```python
from build123d import *

# Parameters (mm, degrees)
F0_W     = 457.2
F0_H     = 914.4
F0_W_2   = 101.6
F0_H_2   = 171.45
F1_DEPTH = 6.35
F2_W     = 381
F2_H     = 38.1
F2_W_2   = 266.7
F2_W_3   = 38.1
F2_H_2   = 187.325
F3_DEPTH = 139.7
F4_W     = 193.675
F4_H     = 6.35
F5_DEPTH = 165.1
F6_W     = 304.8
F6_H     = 254
F7_DEPTH = 12.7
F9_DEPTH = 254
F11_D    = 3.175


with BuildPart() as f1:
    # F0 (on Top) → F1 (new body)
    with BuildSketch(Plane.XY):
        Rectangle(F0_W, F0_H)
        with Locations((133.35, 271.4625)):
            Rectangle(F0_W_2, F0_H_2, mode=Mode.SUBTRACT)
    extrude(amount=F1_DEPTH)

    # F2 (on face) → F3 (join)
    with BuildSketch(Plane(origin=(0, 0, 0), x_dir=(1, 0, 0), z_dir=(0, 0, -1))):
        Polygon((-190.5, 457.2), (-228.6, 457.2), (-228.6, -457.2), (-190.5, -457.2), (-190.5, -419.1), align=None)
        with Locations((0, -438.15)):
            Rectangle(F2_W, F2_H)
        Polygon((190.5, -403.225), (190.5, -419.1), (190.5, -457.2), (228.6, -457.2), (228.6, -368.3), (190.5, -368.3), align=None)
        Polygon((228.6, -174.625), (228.6, 203.2), (190.5, 203.2), (190.5, 165.1), (190.5, -139.7), (190.5, -174.625), align=None)
        with Locations((57.15, 184.15)):
            Rectangle(F2_W_2, F2_H)
        Polygon((28.575, -403.225), (190.5, -403.225), (190.5, -368.3), (190.5, -365.125), (66.675, -365.125), (28.575, -365.125), align=None)
        with Locations((47.625, -271.4625)):
            Rectangle(F2_W_3, F2_H_2)
        Polygon((190.5, -177.8), (190.5, -174.625), (190.5, -139.7), (28.575, -139.7), (28.575, -177.8), (66.675, -177.8), align=None)
    extrude(amount=F3_DEPTH)

    # F4 (on face) → F5 (cut)
    with BuildSketch(Plane.YZ.offset(228.6)):
        with Locations((271.4625, -76.2)):
            Rectangle(F4_W, F4_H)
    extrude(amount=-F5_DEPTH, mode=Mode.SUBTRACT)

    # F6 (on face) → F7 (cut)
    with BuildSketch(Plane.XY.offset(6.35)):
        with Locations((76.2, -330.2)):
            Rectangle(F6_W, F6_H)
    extrude(amount=-F7_DEPTH, mode=Mode.SUBTRACT)

    # F8 (on face) → F9 (join)
    with BuildSketch(Plane.XZ.offset(203.2)):
        Polygon((228.6, -132.720256), (-76.2, 6.35), (-76.2, 0), (-76.2, -0.629744), (228.6, -139.7), align=None)
    extrude(amount=F9_DEPTH)

    # F11 (through all)
    with Locations(Plane.XY.offset(6.35)):
        with Locations((222.25, 336.55), (222.25, 323.85), (222.25, 219.075), (222.25, 206.375)):
            Hole(F11_D / 2)


solid = f1.part
```
Build history of the part. All positions in model axes, mm. A direction names the side the tool comes from. Give positions to 0.01 mm unless a question says otherwise; leave off trailing zeros. Loops run counter-clockwise (first coordinate to the right, second up) from the corner with the lowest first, then second, coordinate; pieces in that order, holes last. Notation, with made-up numbers: (49, -39.75) - (83, -39.75) arc R20 ccw to (83, -31.75) - close; hole circle Ø3 at (52, -29.75). An arc over 180 degrees is marked (long way). Use a Markdown table: item, result.
(1) Wall check: line 1 along Y through (x, z) = (222.25, 3.5); line 2 along X through (y, z) = (336.55, 5); line 3 along Y through (x, z) = (222, 2). Give the ranges that are in metal, low to high.
Taken from the geometry:
| item | result |
|---|---|
| line 1 | -203.2 to 204.79, 207.96 to 217.49, 220.66 to 322.26, 325.44 to 334.96, 338.14 to 457.2 |
| line 2 | -228.6 to 82.55, 184.15 to 220.66, 223.84 to 228.6 |
| line 3 | -203.2 to 204.81, 207.94 to 217.51, 220.64 to 322.28, 325.42 to 334.98, 338.12 to 457.2 |
(2) Band-saw the part on D-D (z = -16.5). Give the cut face in (x, y) (3 decimals), and give its area (3 significant figures).
Taken from the geometry:
| item | result |
|---|---|
| outline | (-228.6, -457.2) - (-190.5, -457.2) - (-190.5, 419.1) - (190.5, 419.1) - (190.5, 403.225) - (28.575, 403.225) - (28.575, 139.7) - (190.5, 139.7) - (190.5, -165.1) - (-76.2, -165.1) - (-76.2, -203.2) - (-41.417, -203.2) - (-41.417, -457.2) - (-26.12, -457.2) - (-26.12, -203.2) - (228.6, -203.2) - (228.6, 174.625) - (190.5, 174.625) - (190.5, 177.8) - (66.675, 177.8) - (66.675, 365.125) - (190.5, 365.125) - (190.5, 368.3) - (228.6, 368.3) - (228.6, 457.2) - (-228.6, 457.2) - close |
| area | 101,000 mm2 |
(3) Pull direction X, two halves, no side cores. Call faces 1 (the face through (66.675, 273, -109)), 2 (the face through (-3, 419.1, -69)), 3 (the face through (-137, -457.2, 4)): +X half, -X half, draft (parallel to the pull), parting line (faces both ways), or undercut.
Taken from the geometry:
| item | result |
|---|---|
| face 1 | +X half |
| face 2 | undercut |
| face 3 | draft |
(4) Drop flat-ended pins along their axis: pin 1 Ø12 at (x, z) = (-150, -73.5) entering from -Y; pin 2 Ø1 at (y, z) = (366, -116.5) entering from +X; pin 3 Ø10 at (x, y) = (95, 101) entering from -Z. Give the stop position or say it passes through.
Taken from the geometry:
| item | result |
|---|---|
| pin 1 | y = 419.1 |
| pin 2 | x = 190.5 |
| pin 3 | z = 0 |
(5) Band-saw the part on B-B (y = 35). Give the cut face in (x, z), and give its area (3 significant figures).
Taken from the geometry:
| item | result |
|---|---|
| outline | (-228.6, -139.7) - (-190.5, -139.7) - (-190.5, 0) - (190.5, 0) - (190.5, -139.7) - (228.6, -139.7) - (228.6, 6.35) - (-228.6, 6.35) - close |
| area | 13,500 mm2 |
(6) Which spindle directions (+Z, -Z, +X, -X, +Y, -Y) get a long thin tool onto all of the face, cutting with end or side? Do faces 4 (the face through (28.575, 270, -69)), 5 (the face through (66, 228, -79.375)), 6 (the face through (78.334, -328.422, -64.159)), 7 (the face through (129, 365.125, -109)), 8 (the face through (6, -203.2, -100)). Say none if no direction does.
Taken from the geometry:
| item | result |
|---|---|
| face 4 | -Z |
| face 5 | +X |
| face 6 | +Z, +X, -Y |
| face 7 | -Z, +X |
| face 8 | -Z, -Y |
(7) Band-saw the part on A-A (y = 271.5). Give the cut face in (x, z) (3 decimals).
Taken from the geometry:
| item | result |
|---|---|
| outline | (-228.6, -139.7) - (-190.5, -139.7) - (-190.5, 0) - (28.575, 0) - (28.575, -139.7) - (66.675, -139.7) - (66.675, -79.375) - (63.5, -79.375) - (63.5, -73.025) - (66.675, -73.025) - (66.675, 0) - (82.55, 0) - (82.55, 6.35) - (-228.6, 6.35) - close; (184.15, 0) - (228.6, 0) - (228.6, 6.35) - (184.15, 6.35) - close |
